Check sheet for the modelled part. Datum: model origin and axes. Units: mm. Face numbers are marked on the shaded views. A direction names the side the tool comes from. Give positions to 0.01 mm unless a question says otherwise; leave off trailing zeros. Order: outer loops, then holes, each group sorted by start corner. A loop starts at its lowest first (then second) coordinate and runs counter-clockwise, first axis right, second up. Notation, with made-up numbers: M 81.5,56 L 89.5,56 A28 ccw 89.5,95 Z; hole C -0.5,75.5 d11. An arc over 180 degrees is marked long. Return JSON: item names as keys, results as strings. Group by question number.
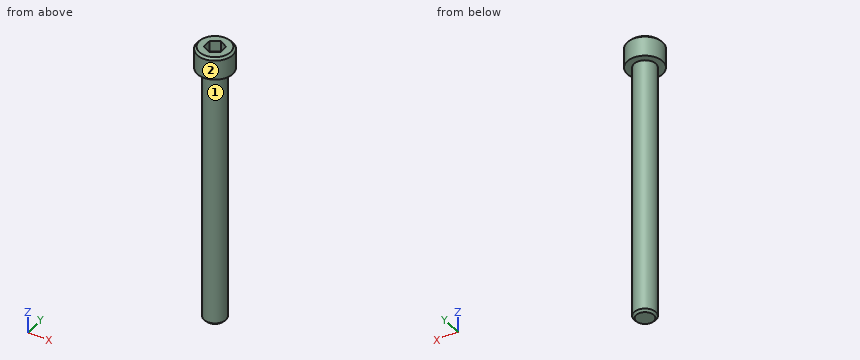
Autodesk Inventor part; units mm, degrees
ref_plane "YZ Plane" through (0, 0, 0) normal (1, 0, 0) x (0, 1, 0)
ref_plane "XZ Plane" through (0, 0, 0) normal (0, 1, 0) x (-1, 0, 0)
ref_plane "XY Plane" through (0, 0, 0) normal (0, 0, 1) x (1, 0, 0)
sketch "Sketch1" plane through (0, 0, 0) normal (0, 0, 1) x (1, 0, 0)
  circle A0 centre (0, 0) radius 4
  dimension "Diameter" = 8
extrude "Extrusion1" add sketch "Sketch1" along normal blind 95
sketch "Sketch2" plane through (0, 0, 95) normal (0, 0, 1) x (1, 0, 0)
  circle A0 centre (0, 0) radius 4
  circle A1 centre (0, 0) radius 6.5
  dimension "Head_Diameter" = 13
extrude "Extrusion2" add sketch "Sketch2" along normal blind 8 contours A0 | A1
sketch "Sketch3" plane through (0, 0, 103) normal (0, 0, 1) x (1, 0, 0)
  circle A0 centre (0, 0) radius 6.5
  circle A1 centre (0, 0) radius 3.4641 construction
  line L0 (0, 3.4641) -> (3, 1.7321)
  line L1 (3, -1.7321) -> (3, 1.7321)
  line L2 (0, 3.4641) -> (-3, 1.7321)
  line L3 (-3, -1.7321) -> (-3, 1.7321)
  line L4 (-3, -1.7321) -> (0, -3.4641)
  line L5 (3, -1.7321) -> (0, -3.4641)
  dimension "Hex_Width" = 6
extrude "Extrusion3" cut sketch "Sketch3" against normal blind 4 contours L0 L1 L5 L4 L3 L2
thread "Thread1"
chamfer "Chamfer1" distance 0.8 angle 45 2 edges at (-6.5, 0, 103) (-4, 0, 0)
equation "\"d9\" = ThreadLength"
equation "\"d12\" = Chamfer"
equation "\"ThreadLength\" = 28"
properties part number "SCREW, SOCKET HD, P, 12.9, M8X1.25X95MM"
1) Sectioned sample at B-B on z = 41. Record the boundary of the cut face in (x, y).
2) Sectioned sample at A-A on y = 0. Record the boundary of the cut face in (x, z).
3) Material ranges on line 1 along Z through (x, y) = (-4.25, 3.5); line 2 along Z through (x, y) = (1.5, 1); line 3 along X through (y, z) = (-1, 14), recorded low to high.
4) Tool access check on the marked faces 1 and 2. Record the directions out of +Z, -Z, +X, -X, +Y, -Y that give a thin tool (end or side, any length) a straight path to the whole face; none if there is none.
5) Depth check by flat-ended pin: P1, Ø1.5, axis at x = -1, y = 5, coming from the -Z side; P2, Ø6.5, axis at x = -2, y = 1, coming from the -Z side; P3, Ø2, axis at x = 4, z = 76, coming from the +Y side; P4, Ø1.5, axis at x = -1, y = -4.5, coming from the -Z side. Enter the tip coordinate at first touch or a pass-through.
Reply:
{
 "1": {"outline": "C 0,0 d8"},
 "2": {"outline": "M -6.5,95 L -4,95 L -4,0.8 L -3.2,0 L 3.2,0 L 4,0.8 L 4,95 L 6.5,95 L 6.5,102.2 L 5.7,103 L 3,103 L 3,99 L -3,99 L -3,103 L -5.7,103 L -6.5,102.2 Z"},
 "3": {"line 1": "95 to 103", "line 2": "0 to 99", "line 3": "-3.87 to 3.87"},
 "4": {"face 1": "-Z", "face 2": "+Z, -Z"},
 "5": {"P1": "z = 95", "P2": "z = 0", "P3": "y = 2.65", "P4": "z = 0.66"}
}
